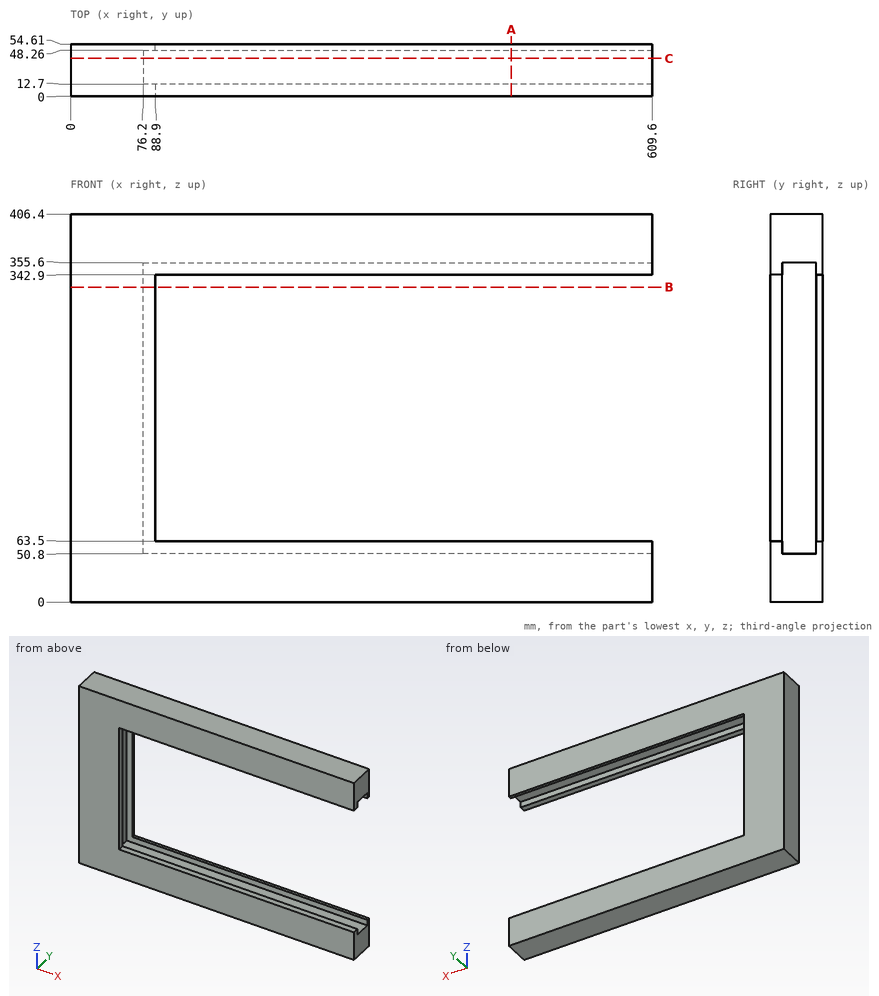
Part print with two shaded views. Sizes in mm from the minimum x, y, z corner. Round coordinates to 2 decimals unless told otherwise and drop trailing zeros. Loops run counter-clockwise (first coordinate to the right, second up) from the corner with the lowest first, then second, coordinate; pieces in that order, holes last. Notation, with made-up numbers: M -15,29.25 L -1,29.25 A25 ccw -1,41.25 Z; hole C 54,83 d9. An arc over 180 degrees is marked long. Put each result on its own line as item: value. Start each with the question number.
Item 1: Cut at A-A (x = 462). List the corners of the cut face in (y, z), then the cut area to 3 significant figures.
Item 2: Cut at C-C (y = 39.5). List the corners of the cut face in (x, z), then the cut area to 3 significant figures.
Item 3: Drill centre lines: line 1 along Z through (x, y) = (122, 4); line 2 along Z through (x, y) = (306, 17.5); line 3 along Y through (x, z) = (88.5, 71.5). Where is each one in solid material? Low to high.
Item 4: Drop flat-ended pins along their axis: P1, Ø10, axis at y = 14.5, z = 326, coming from the +X side; P2, Ø10.5, axis at y = 28, z = 247, coming from the +X side. Give the stop position or say it passes through.
Item 5: Cut at B-B (z = 330). List the corners of the cut face in (x, y).
Answer block:
1. outline: M 0,0 L 54.61,0 L 54.61,63.5 L 48.26,63.5 L 48.26,50.8 L 12.7,50.8 L 12.7,63.5 L 0,63.5 Z; M 0,342.9 L 12.7,342.9 L 12.7,355.6 L 48.26,355.6 L 48.26,342.9 L 54.61,342.9 L 54.61,406.4 L 0,406.4 Z
1. area: 6,030 mm2
2. outline: M 0,0 L 609.6,0 L 609.6,50.8 L 76.2,50.8 L 76.2,355.6 L 609.6,355.6 L 609.6,406.4 L 0,406.4 Z
2. area: 85,200 mm2
3. line 1: 0 to 63.5, 342.9 to 406.4
3. line 2: 0 to 50.8, 355.6 to 406.4
3. line 3: 0 to 12.7, 48.26 to 54.61
4. P1: x = 88.9
4. P2: x = 76.2
5. outline: M 0,0 L 88.9,0 L 88.9,12.7 L 76.2,12.7 L 76.2,48.26 L 88.9,48.26 L 88.9,54.61 L 0,54.61 Z
